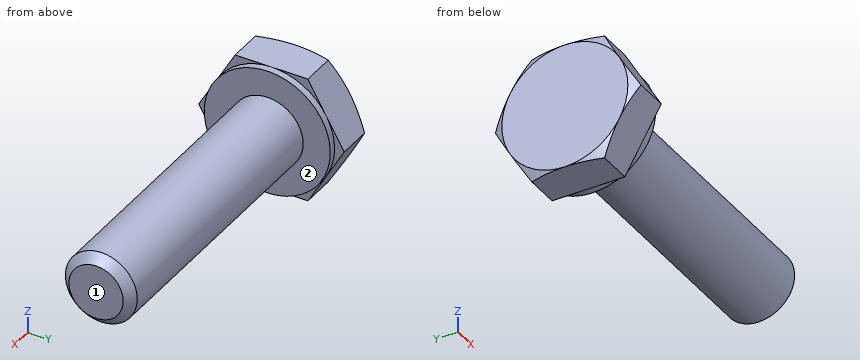
Autodesk Inventor part; units mm, degrees
ref_plane "Work Plane1" through (1.525, 0, 0) normal (0, 0, 1) x (1, 0, 0)
ref_plane "YZ Plane" through (0, 0, 0) normal (1, 0, 0) x (0, 1, 0)
ref_plane "XZ Plane" through (0, 0, 0) normal (0, 1, 0) x (-1, 0, 0)
sketch "Sketch1" plane through (0, 0, 0) normal (0, 0, 1) x (1, 0, 0)
  line L0 (0, 5.5626) -> (0, 3.175)
  line L1 (10.414, 3.175) -> (25.4, 3.175)
  line L2 (25.4, 3.175) -> (25.4, 0)
  line L3 (25.4, 0) -> (-0.6351, 0)
  line L4 (-5.8421, 0) -> (30.607, 0)
  line L5 (-0.6351, 0) -> (-0.6351, 5.5626)
  line L6 (-0.6351, 5.5626) -> (0, 5.5626)
  line L7 (10.414, 3.175) -> (0.2539, 3.175)
  line L8 (0.2539, 3.175) -> (0, 3.175)
  line L9 (0, -1.1125) -> (0, 6.6751)
  dimension "d0" = 25.4
  dimension "d1" = 14.986
  dimension "d2" = 6.35
  dimension "d9" = 0.6351
  dimension "d10" = 11.1252
  dimension "d13" = 10.1601
  dimension "d14" = 6.35
revolve "Body" add sketch "Sketch1" angle 360 about axis through (25.4, 0, 0) along (-1, 0, 0)
sketch "Sketch2" plane through (-0.6351, 0, 0) normal (-1, 0, 0) x (0, 0, 1)
  line L0 (0, 6.4231) -> (5.5626, 3.2116)
  line L1 (5.5626, 3.2116) -> (5.5626, -3.2116)
  line L2 (5.5626, -3.2116) -> (0, -6.4231)
  line L3 (0, -6.4231) -> (-5.5626, -3.2116)
  line L4 (-5.5626, -3.2116) -> (-5.5626, 3.2116)
  line L5 (-5.5626, 3.2116) -> (0, 6.4231)
  point P0 (0, 0)
  point P1 (0, 0)
  dimension "d11" = 11.1252
extrude "Head" add sketch "Sketch2" along normal blind 3.5052
sketch "Sketch4" plane through (0, 0, 0) normal (0, 0, 1) x (1, 0, 0)
  line L0 (-4.1403, 5.5626) -> (-4.1403, 6.4231)
  line L1 (-4.1403, 6.4231) -> (-3.6435, 6.4231)
  line L2 (-3.6435, 6.4231) -> (-4.1403, 5.5626)
  line L3 (-4.8413, 0) -> (0.0659, 0)
  line L4 (-0.6351, 6.4231) -> (-4.1403, 6.4231)
  line L5 (-4.1403, 3.2116) -> (-4.1403, 6.4231)
  dimension "d5" = 30
  dimension "d19" = 11.1252
revolve "Chamfer1" cut sketch "Sketch4" angle 360 about axis through (-10, 0, 0) along (1, 0, 0)
thread "Thread"
chamfer "Chamfer2" distance 0.779 distance2 0.7791 1 edges at (25.4, -3.175, 0) measured on face at (25.4, -0.1276, -1.0506)
ref_plane "Work Plane1" through (1.525, 0, 0) normal (0, 0, 1) x (1, 0, 0)
equation "\"d0\" = NLG"
equation "\"d1\" = GEL"
equation "\"d2\" = GD"
equation "\"d10\" = SD2"
equation "\"d14\" = BDM"
equation "\"d11\" = SW"
equation "\"d3\" = KOH - SD"
equation "\"d5\" = ANG1"
equation "\"d19\" = SW0"
equation "\"d15\" = GEL"
equation "\"d6\" = -0.5 * SPD + 0.5 * GD"
equation "\"NLG\" = 25.4"
equation "\"GD\" = 6.35"
equation "\"BDM\" = 6.35"
equation "\"KOH\" = 4.1402"
equation "\"GEL\" = 14.986"
equation "\"SW\" = 11.1252"
equation "\"SW0\" = SW"
equation "\"SPD\" = GD1"
equation "\"SD2\" = SW"
equation "\"SD\" = 0.635"
equation "\"ANG1\" = 30deg"
equation "\"GAL\" = 10.16"
equation "\"GUL\" = 0.77902"
equation "\"RR\" = 0.381"
equation "\"WFT\" = SD"
equation "\"GD1\" = 4.79196"
equation "\"THREADDIA\" = 6.35"
equation "\"SDH\" = SW"
equation "\"SDHG\" = 0.254"
equation "\"TOA\" = 30deg"
equation "\"FAWI\" = 45deg"
equation "\"NND\" = 6.35"
equation "\"E0\" = 12.84961"
properties part number "AS 2465 - 1/4 x 1  UNC" material "Steel, Mild"
Design review of the part built by this model. Coordinates are the model's own, in mm. Face numbers are marked on the shaded views. A direction names the side the tool comes from. Coordinates: 2 decimals unless noted, no trailing zeros. Write each loop counter-clockwise with the first axis right and the second up, starting at its lowest first coordinate (ties: lowest second). Pieces come first, ordered by that corner, then holes.
1) Add section A-A (x = -2). Write out the cut boundary in (y, z).
2) Machinability: for the marked faces 1 and 2, which of the approach directions +Z, -Z, +X, -X, +Y, -Y give a long, thin tool a straight path to every point of the face, cutting with its end or side? Answer none if there is none.
3) Insertion check: pin 1 (1.4 mm diameter, centred on y = 3.5, z = -5, fed in from +X); pin 2 (1.5 mm diameter, centred on x = 20.5, y = -4.5, fed in from +Z); pin 3 (1.5 mm diameter, centred on x = 16.5, y = 3.5, fed in from -Z); pin 4 (1.5 mm diameter, centred on x = 5, z = 3, fed in from -Y). Each pin has a flat end and moves straight along its axis. Give the tip position at first contact, or say it passes through.
4) Add section B-B (x = 16.25). Write out the cut boundary in (y, z) (3 decimals), plus the area to 3 significant figures.
5) To check wall thickness, follow L1, parallel to X at y = -2.25, z = 4.5; L2, parallel to Y at x = 20.75, z = 0 (3 decimals); L3, parallel to Y at x = -0.75, z = 1.25. State the ranges of each line that lie inside material, in increasing order.
Check result:
1. outline: (-6.42, 0) - (-3.21, -5.56) - (3.21, -5.56) - (6.42, 0) - (3.21, 5.56) - (-3.21, 5.56) - close
2. face 1: +Z, -Z, +X, +Y, -Y
2. face 2: +X
3. pin 1: stops at x = 0
3. pin 2: passes through
3. pin 3: stops at z = -1.59
3. pin 4: stops at y = -2.24
4. outline: circle Ø6.35 at (0, 0)
4. area: 31.7 mm2
5. L1: x = -4.14 to 0
5. L2: y = -3.175 to 3.175
5. L3: y = -5.7 to 5.7
